Part model, mm, in its own coordinate system. Coordinates: 2 decimals unless noted, no trailing zeros. Write each loop counter-clockwise with the first axis right and the second up, starting at its lowest first coordinate (ties: lowest second). Pieces come first, ordered by that corner, then holes. Notation, with made-up numbers: (3.5, -18) - (17.5, -18) arc R18 cw to (17.5, 2) - close; hole circle Ø10 at (-19, 16). An arc over 180 degrees is marked (long way). Write each question's results on one line, items separated by ' | '.
from build123d import *

# Parameters (mm, degrees)
SKETCH1_W           = 834.8
SKETCH1_H           = 471.91
BOSS_EXTRUDE1_DEPTH = 10
SKETCH2_R           = 5


with BuildPart() as part:
    # Sketch1 → Boss-Extrude1 (new body)
    with BuildSketch(Plane(origin=(0, 0, 0), x_dir=(0, 0, -1), z_dir=(1, 0, 0))):
        Rectangle(SKETCH1_W, SKETCH1_H)
    extrude(amount=BOSS_EXTRUDE1_DEPTH)

    # Sweep1: sweep along a curve in space
    with BuildLine() as sweep1_path:
        Line((10, -210, -50), (40, -210, -50))
        Line((40, -210, -50), (40, -210, 50))
        Line((10, -210, 50), (40, -210, 50))
    # Sketch2 → Sweep1 (sweep)
    with BuildSketch(Plane(origin=(10, 0, 0), x_dir=(0, 0, -1), z_dir=(1, 0, 0))):
        with Locations((50, -210)):
            Circle(SKETCH2_R)
    sweep(path=sweep1_path.line, transition=Transition.RIGHT)


solid = part.part
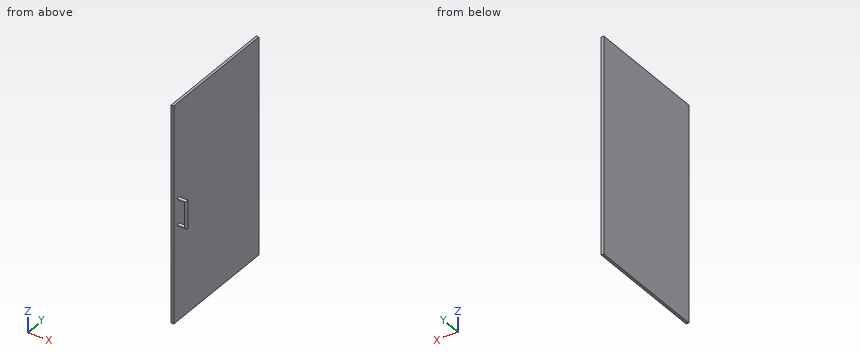
(1) Flat gauge pin, fed straight in: P1, Ø8, axis at x = 10.5, y = -42.5, coming from the -Z side. Where does the tip first touch, or does it go through?
Return value:
P1: stops at z = -417.4
(2) Saw through at A-A on z = -0.5. Write the cut outline in (x, y) (3 decimals).
Return value:
outline: (0, -235.955) - (10, -235.955) - (10, 235.955) - (0, 235.955) - close; circle Ø10 at (40, -210)
(3) Saw through at B-B on x = 17.5. Write the cut outline in (y, z), then the cut area to 3 significant figures.
Return value:
outline: circle Ø10 at (-210, -50); circle Ø10 at (-210, 50) | area: 157 mm^2
(4) Wall check: line 1 (X direction, y = -164.5, z = -20); line 2 (Y direction, x = 22.5, z = 48.5). Give the ranges that are in metal, low to high. Write a range as from..to.
Return value:
line 1: x = 0..10 | line 2: y = -214.77..-205.23
(5) Saw through at D-D on z = 151. Write the cut outline in (x, y) (3 decimals).
Return value:
outline: (0, -235.955) - (10, -235.955) - (10, 235.955) - (0, 235.955) - close
(6) Saw through at C-C on y = -69. Write the cut outline in (x, z).
Return value:
outline: (0, -417.4) - (10, -417.4) - (10, 417.4) - (0, 417.4) - close
